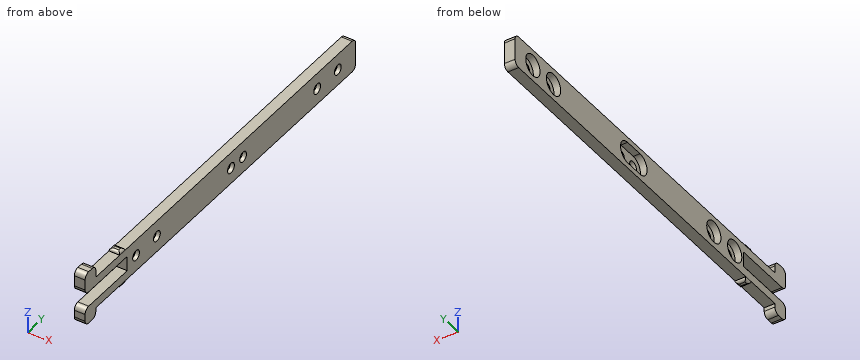
```python
from build123d import *

# Parameters (mm, degrees)
SKETCH062_R             = 1.9
PAD020_DEPTH            = 4
SKETCH063_R             = 4
POCKET042_DEPTH         = 2.5
FILLET015_R             = 2
FILLET016_R             = 1
FILLET017_R             = 2
BODY016_PLACEMENT_ANGLE = 270


with BuildPart() as part:
    # Sketch062 → Pad020 (new body)
    with BuildSketch(Plane.XZ):
        Polygon((4, 0), (-125.535636, 0), (-125.535636, -1.01), (-128.535636, -1.01), (-128.535636, 0), (-141.91974, 0), (-141.91974, -3.395505), (-147.91974, -3.395505), (-147.91974, 3.2), (-124.257385, 3.2), (-124.257385, 8.8), (-147.91974, 8.8), (-147.91974, 16.699631), (-141.91974, 16.699631), (-141.91974, 12), (-128.535636, 12), (-128.535636, 13.01), (-125.535636, 13.01), (-125.535636, 12), (4, 12), align=None)
        with Locations((-66, 6)):
            Circle(SKETCH062_R, mode=Mode.SUBTRACT)
        with Locations((-6, 6)):
            Circle(SKETCH062_R, mode=Mode.SUBTRACT)
        with Locations((-107.6, 6)):
            Circle(SKETCH062_R, mode=Mode.SUBTRACT)
        with Locations((-17.6, 6)):
            Circle(SKETCH062_R, mode=Mode.SUBTRACT)
        with Locations((-59.2, 6)):
            Circle(SKETCH062_R, mode=Mode.SUBTRACT)
        with Locations((-119.3, 6)):
            Circle(SKETCH062_R, mode=Mode.SUBTRACT)
    extrude(amount=PAD020_DEPTH)

    # Sketch063 (on Face27 of Pad020) → Pocket042 (cut)
    with BuildSketch(Plane(origin=(0, 0, 0), x_dir=(1, 0, 0), z_dir=(0, 1, 0))):
        with Locations((-107.6, -6)):
            Circle(SKETCH063_R)
        with Locations((-6, -6)):
            Circle(SKETCH063_R)
        with Locations((-17.6, -6)):
            Circle(SKETCH063_R)
        with Locations((-119.3, -6)):
            Circle(SKETCH063_R)
        with BuildLine():
            ThreePointArc((-66.1179939879, -2), (-70.1179939879, -6), (-66.1179939879, -10))
            Line((-66.1179939879, -10), (-59.2, -10))
            ThreePointArc((-59.2, -10), (-55.2, -6), (-59.2, -2))
            Line((-66.1179939879, -2), (-59.2, -2))
        make_face()
    extrude(amount=-POCKET042_DEPTH, mode=Mode.SUBTRACT)

    # Fillet015
    fillet015_edges = [part.edges().sort_by_distance(p)[0] for p in [
        (4, -2, 12),
        (4, -2, 0),
    ]]
    fillet(fillet015_edges, radius=FILLET015_R)

    # Fillet016
    fillet016_edges = [part.edges().sort_by_distance(p)[0] for p in [
        (-125.535636, -2, -1.01),
        (-128.535636, -2, -1.01),
        (-127.035636, 0, -1.01),
        (-127.035636, -4, -1.01),
        (-128.535636, -2, 13.01),
        (-125.535636, -2, 13.01),
        (-127.035636, 0, 13.01),
        (-127.035636, -4, 13.01),
    ]]
    fillet(fillet016_edges, radius=FILLET016_R)

    # Fillet017
    fillet017_edges = [part.edges().sort_by_distance(p)[0] for p in [
        (-141.91974, -2, 16.699631),
        (-147.91974, -2, 16.699631),
        (-147.91974, -2, 8.8),
        (-147.91974, -2, 3.2),
        (-147.91974, -2, -3.395505),
        (-141.91974, -2, -3.395505),
    ]]
    fillet(fillet017_edges, radius=FILLET017_R)


with BuildPart() as part_1:
    # Body016 placement: moved
    add(part.part.moved(Location((8.5, 121, 40.5))).rotate(Axis((8.5, 121, 40.5), (0, 0, -1)), BODY016_PLACEMENT_ANGLE))


solid = part_1.part
```
Source: CAD feature listing. Evaluate the final solid. Frame: model axes, mm. Coordinates: 2 decimals unless noted, no trailing zeros. Order: outer loops, then holes, each group sorted by start corner. A loop starts at its lowest first (then second) coordinate and runs counter-clockwise, first axis right, second up. Notation, with made-up numbers: M 59.25,-37 L 117.25,-37 A6 ccw 117.25,-28 Z; hole C 21.25,8 d8. An arc over 180 degrees is marked long. Write each question's results on one line, items separated by ' | '. Start each with the question number.
1) Line query: line 1 (Y direction, x = 10.15, z = 46.5); line 2 (Z direction, x = 11.55, y = 103.4); line 3 (Z direction, x = 9.8, y = 61). Output: solid intervals per line, ascending. Write a range as from..to.
2) Section query C-C (y = 76.5). Return the cut outline in (x, z).
3) Contact query for flat-ended pins moving along their axis: pin 1 Ø2 at (x, z) = (10.5, 45.5) entering from -Y; pin 2 Ø0.8 at (x, y) = (9.5, 59) entering from -Z; pin 3 Ø1.2 at (x, y) = (11, -10) entering from +Z. Output: stop coordinate, or through.
4) Section query B-B (y = -15.5). Return the cut outline in (x, z), plus the area to 3 significant figures.
5) Section query A-A (y = 115). Return the cut outline in (x, z).
Answers:
1) line 1: y = -3.26..-2.3, 5.7..9.4, 17.4..50.88, 65.8..99.4, 107.4..111, 119..125 | line 2: z = 40.5..44.6, 48.4..52.5 | line 3: z = 40.5..42.5, 50.5..52.5
2) outline: M 8.5,40.5 L 12.5,40.5 L 12.5,52.5 L 8.5,52.5 Z
3) pin 1: stops at y = -3.26 | pin 2: stops at z = 40.5 | pin 3: stops at z = 52.5
4) outline: M 8.5,40.5 L 12.5,40.5 L 12.5,43.7 L 8.5,43.7 Z; M 8.5,49.3 L 12.5,49.3 L 12.5,52.5 L 8.5,52.5 Z | area: 25.6 mm^2
5) outline: M 8.5,40.5 L 12.5,40.5 L 12.5,44.6 L 11,44.6 L 11,42.5 L 8.5,42.5 Z; M 8.5,50.5 L 11,50.5 L 11,48.4 L 12.5,48.4 L 12.5,52.5 L 8.5,52.5 Z
